Could you check a few things on this model? Use its own coordinates, in mm. Face numbers are marked on the shaded views. A direction names the side the tool comes from. Give positions to 0.01 mm unless a question says otherwise; leave off trailing zeros. Loops run counter-clockwise (first coordinate to the right, second up) from the corner with the lowest first, then second, coordinate; pieces in that order, holes last. Notation, with made-up numbers: (-32.75, 9.25) - (-26.75, 9.25) arc R24 ccw to (-26.75, 46.25) - close; hole circle Ø1 at (-12.5, 23). An arc over 180 degrees is marked (long way). One line per item, written item: value. Start each with the question number.
Q1. For the marked faces 1 and 2, which set-ups out of +Z, -Z, +X, -X, +Y, -Y let a thin tool reach every point of the face, with its end or its side?
Q2. If I drill on line 1 (X direction, y = 15.25, z = 7); line 2 (X direction, y = 11, z = 8.5); line 3 (Y direction, x = 8.25, z = 42), over which ranges is the centre line in solid material (lowest first)? Write a range as from..to.
Q3. I want a section at B-B (x = 9.45). Please give me the cut outline in (y, z), then the cut area to 3 significant figures.
Q4. If we mould it in two halves opening along X, with no side actions, what happens to the marked faces 3, 4 and 5? For each: released by +X, released by -X, zero draft, split by the parting line, or undercut.
Q5. I want a section at C-C (z = 43.5). Please give me the cut outline in (x, y).
Q6. I want a section at A-A (y = 13.25). Please give me the cut outline in (x, z).
```python
from build123d import *

# Parameters (mm, degrees)
EXTRUDE_1_DEPTH = 48
FILLET_1_R      = 0.5
FILLET_2_R      = 0.5


with BuildPart() as part:
    # Эскиз1 → Бобышка-Вытянуть1 (new body)
    with BuildSketch(Plane.XY):
        with BuildLine():
            Line((0.7, 3.35), (18.2, 3.35))
            ThreePointArc((18.2, 3.35), (18.553553391, 3.496446609), (18.7, 3.85))
            Line((18.7, 3.85), (18.7, 25.85))
            ThreePointArc((18.7, 25.85), (18.553553391, 26.203553391), (18.2, 26.35))
            Line((18.2, 26.35), (0.7, 26.35))
            ThreePointArc((0.7, 26.35), (0.346446609, 26.203553391), (0.2, 25.85))
            Line((0.2, 25.85), (0.2, 3.85))
            ThreePointArc((0.2, 3.85), (0.346446609, 3.496446609), (0.7, 3.35))
        make_face()
        with BuildLine():
            Line((6.75, 17.55), (6.75, 12.15))
            ThreePointArc((6.75, 12.15), (9.45, 9.45), (12.15, 12.15))
            Line((12.15, 12.15), (12.15, 17.55))
            ThreePointArc((12.15, 17.55), (9.45, 20.25), (6.75, 17.55))
        make_face(mode=Mode.SUBTRACT)
    extrude(amount=EXTRUDE_1_DEPTH)

    # Скругление1
    fillet_1_edges = [part.edges().sort_by_distance(p)[0] for p in [
        (9.45, 3.35, 0),
        (0.346446609, 3.496446609, 0),
        (0.2, 14.85, 0),
        (0.346446609, 26.203553391, 0),
        (9.45, 20.25, 0),
        (6.75, 14.85, 0),
        (9.45, 9.45, 0),
        (12.15, 14.85, 0),
        (9.45, 26.35, 0),
        (18.553553391, 26.203553391, 0),
        (18.7, 14.85, 0),
        (18.553553391, 3.496446609, 0),
    ]]
    fillet(fillet_1_edges, radius=FILLET_1_R)

    # Скругление2
    fillet_2_edges = [part.edges().sort_by_distance(p)[0] for p in [
        (0.346446609, 3.496446609, 48),
        (9.45, 3.35, 48),
        (18.553553391, 3.496446609, 48),
        (18.7, 14.85, 48),
        (9.45, 20.25, 48),
        (6.75, 14.85, 48),
        (9.45, 9.45, 48),
        (12.15, 14.85, 48),
        (18.553553391, 26.203553391, 48),
        (9.45, 26.35, 48),
        (0.346446609, 26.203553391, 48),
        (0.2, 14.85, 48),
    ]]
    fillet(fillet_2_edges, radius=FILLET_2_R)


solid = part.part
```
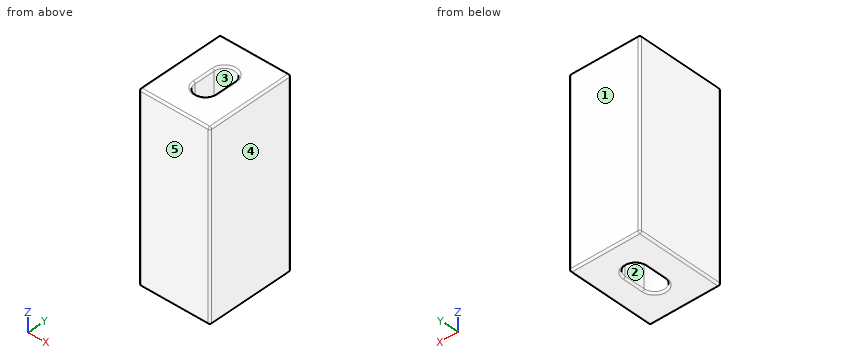
Worked answers:
1. face 1: +Z, -Z, +X, -X, +Y
1. face 2: +Z, -Z
2. line 1: x = 0.2..6.75, 12.15..18.7
2. line 2: x = 0.2..7.01, 11.89..18.7
2. line 3: y = 3.35..9.73, 19.97..26.35
3. outline: (3.35, 0.5) arc R0.5 ccw to (3.85, 0) - (8.95, 0) arc R0.5 ccw to (9.45, 0.5) - (9.45, 47.5) arc R0.5 ccw to (8.95, 48) - (3.85, 48) arc R0.5 ccw to (3.35, 47.5) - close; (20.25, 0.5) arc R0.5 ccw to (20.75, 0) - (25.85, 0) arc R0.5 ccw to (26.35, 0.5) - (26.35, 47.5) arc R0.5 ccw to (25.85, 48) - (20.75, 48) arc R0.5 ccw to (20.25, 47.5) - close
3. area: 585 mm²
4. face 3: undercut
4. face 4: released by +X
4. face 5: zero draft
5. outline: (0.2, 3.85) arc R0.5 ccw to (0.7, 3.35) - (18.2, 3.35) arc R0.5 ccw to (18.7, 3.85) - (18.7, 25.85) arc R0.5 ccw to (18.2, 26.35) - (0.7, 26.35) arc R0.5 ccw to (0.2, 25.85) - close; hole (6.75, 12.15) arc R2.7 ccw to (12.15, 12.15) - (12.15, 17.55) arc R2.7 ccw to (6.75, 17.55) - close
6. outline: (0.2, 0.5) arc R0.5 ccw to (0.7, 0) - (6.25, 0) arc R0.5 ccw to (6.75, 0.5) - (6.75, 47.5) arc R0.5 ccw to (6.25, 48) - (0.7, 48) arc R0.5 ccw to (0.2, 47.5) - close; (12.15, 0.5) arc R0.5 ccw to (12.65, 0) - (18.2, 0) arc R0.5 ccw to (18.7, 0.5) - (18.7, 47.5) arc R0.5 ccw to (18.2, 48) - (12.65, 48) arc R0.5 ccw to (12.15, 47.5) - close
